Input: part model. Units: mm. Frame: model coordinates. Face numbers are marked on the shaded views. A direction names the side the tool comes from. Give positions to 0.01 mm unless a question says otherwise; leave off trailing zeros. Loops run counter-clockwise (first coordinate to the right, second up) from the corner with the lowest first, then second, coordinate; pieces in that order, holes last. Notation, with made-up numbers: (66.25, 61) -> (75.25, 61) arc R18 cw to (75.25, 74) -> close; hole circle Ø4 at (-26, 22). An arc over 180 degrees is marked (long way). Answer as a JSON object with one key per item and string values.
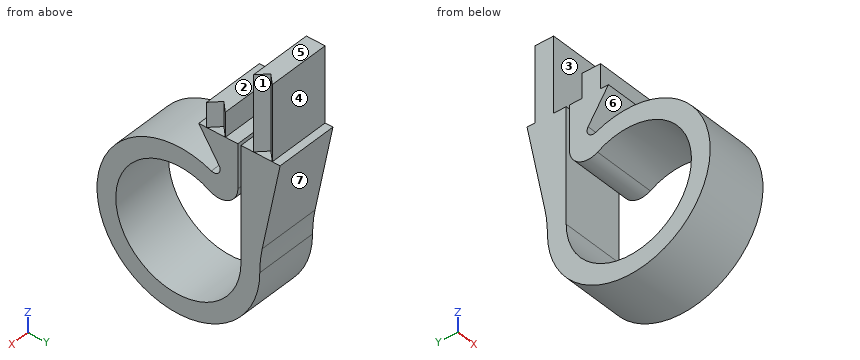
```python
from build123d import *

# Parameters (mm, degrees)
BOSS_EXTRUDE1_DEPTH = 10
BOSS_EXTRUDE4_DEPTH = 12
SKETCH6_W           = 8.1
SKETCH6_H           = 3
CUT_EXTRUDE2_DEPTH  = 12


with BuildPart() as part:
    # Sketch1 → Boss-Extrude1 (new body)
    with BuildSketch(Plane(origin=(0, 0, 0), x_dir=(0, 0, -1), z_dir=(1, 0, 0))):
        with BuildLine():
            Line((-11.258330249, -0.5), (-18.258330249, -0.5))
            Line((-18.258330249, -0.5), (-18.258330249, -6.75))
            Line((-18.258330249, -6.75), (-13.354440804, -3.5))
            ThreePointArc((-13.354440804, -3.5), (-12.156943399, -3.569431047), (-11.887579875, -4.738304007))
            ThreePointArc((-11.887579875, -4.738304007), (7.092177102, -20.894999952), (0, 3))
            ThreePointArc((0, 3), (-1.967023285, 3.096964568), (-3.914973414, 3.38691806))
            Line((-3.914973414, 3.38691806), (-18.258330249, 6.25))
            Line((-18.258330249, 6.25), (-18.258330249, 0))
            Line((-18.258330249, 0), (0, 0))
            ThreePointArc((0, 0), (5, -18.660254038), (-8.660254038, -5))
            ThreePointArc((-8.660254038, -5), (-8.660254038, -2), (-11.258330249, -0.5))
        make_face()
    extrude(amount=BOSS_EXTRUDE1_DEPTH)

    # Sketch2 → Boss-Extrude4 (add)
    with BuildSketch(Plane.XY.offset(18.258330249)):
        Polygon((0, 2), (10, 2), (8.5, 3.5), (10, 5), (0, 5), align=None)
        Polygon((0, -5.5), (10, -5.5), (8.5, -4), (10, -2.5), (0, -2.5), align=None)
    extrude(amount=BOSS_EXTRUDE4_DEPTH)

    # Sketch6 → Cut-Extrude2 (cut)
    with BuildSketch(Plane.ZY):
        with Locations((26.208330249, -4)):
            Rectangle(SKETCH6_W, SKETCH6_H)
    extrude(amount=-CUT_EXTRUDE2_DEPTH, mode=Mode.SUBTRACT)


solid = part.part
```
Q1. Access query for the marked faces 1, 2 and 3. Directions: +Z, -Z, +X, -X, +Y, -Y. A direction counts if a zero-diameter tool reaches every point of the face in a straight line with its end or side. Return the directions, or none.
Evaluation:
{"face 1": "+Z, +X", "face 2": "+Z, +X, -X, -Y", "face 3": "+Z, +X, -X"}
Q2. Section C-C, the plane y = -6.25. Return the cut outline in (x, z).
Evaluation:
{"outline": "(0, -12.45) -> (10, -12.45) -> (10, -9.27) -> (0, -9.27) -> close; (0, 9.27) -> (10, 9.27) -> (10, 12.45) -> (0, 12.45) -> close; (0, 17.5) -> (10, 17.5) -> (10, 18.26) -> (0, 18.26) -> close"}
Q3. Draft query along Z for the marked faces 4, 5, 6 and 7. Return one class per face: +Z half, -Z half, draft (parallel to the pull), parting line (faces both ways), or undercut.
Evaluation:
{"face 4": "draft", "face 5": "+Z half", "face 6": "undercut", "face 7": "-Z half"}
Q4. Pin query (flat end, axial travel): pin 1 (1.5 mm diameter, centred on x = 2.5, z = 22, fed in from -Y); pin 2 (4.5 mm diameter, centred on x = 3, z = 21, fed in from +Y); pin 3 (2 mm diameter, centred on x = 6.5, z = 15.5, fed in from +Y). Return the tip coordinate at first contact, or that it passes through.
Evaluation:
{"pin 1": "stops at y = -5.5", "pin 2": "stops at y = 5", "pin 3": "stops at y = 5.9"}
Q5. Ray query, line 1 along Z through (x, y) = (1.25, -3.5); line 2 along Z through (x, y) = (7.25, -10); line 3 along Y through (x, z) = (9.5, 9). Return the intervals inside material, ascending.
Evaluation:
{"line 1": "z = -11.26 to -7.6, 8.26 to 12.25, 13.35 to 22.16", "line 2": "z = -13 to -10, 10 to 13", "line 3": "y = -19.38 to -14.36, -5.64 to -1.53, 0 to 4.4"}
Q6. Section B-B, the plane z = 3. Return the cut outline in (x, y), then the cut area to 3 significant figures.
Evaluation:
{"outline": "(0, -22.65) -> (10, -22.65) -> (10, -19.54) -> (0, -19.54) -> close; (0, 0) -> (10, 0) -> (10, 3.23) -> (0, 3.23) -> close", "area": "63.4 mm2"}
Q7. Section A-A, the plane y = -10. Return the cut outline in (x, z), then the cut area to 3 significant figures.
Evaluation:
{"outline": "(0, -13) -> (10, -13) -> (10, -10) -> (0, -10) -> close; (0, 10) -> (10, 10) -> (10, 13) -> (0, 13) -> close", "area": "60.0 mm2"}
Q8. Section D-D, the plane x = 2.75. Return the cut outline in (y, z).
Evaluation:
{"outline": "(-6.75, 18.26) -> (-3.5, 13.35) arc R1 cw to (-4.74, 11.89) arc R13 ccw (long way) to (3, 0) arc R20 cw to (3.39, 3.91) -> (6.25, 18.26) -> (5, 18.26) -> (5, 30.26) -> (2, 30.26) -> (2, 18.26) -> (0, 18.26) -> (0, 0) arc R10 cw (long way) to (-5, 8.66) arc R3 ccw to (-0.5, 11.26) -> (-0.5, 18.26) -> (-2.5, 18.26) -> (-2.5, 22.16) -> (-5.5, 22.16) -> (-5.5, 18.26) -> close"}
